Could you check a few things on this model? Use its own coordinates, in mm. Face numbers are marked on the shaded views. A direction names the side the tool comes from. Coordinates: 2 decimals unless noted, no trailing zeros. Loops run counter-clockwise (first coordinate to the right, second up) from the corner with the lowest first, then second, coordinate; pieces in that order, holes last. Notation, with made-up numbers: (13, -24.75) -> (24, -24.75) arc R23 cw to (24, 1.25) -> close; hole circle Ø1 at (86.25, 65.25). An arc over 180 degrees is marked (long way). One line per question, with ' | ' between items.
```python
from build123d import *

# Parameters (mm, degrees)
ESQUISSE1_R             = 16
BOSS_EXTRU_1_DEPTH      = 36.4
ESQUISSE2_R             = 9.5
BOSS_EXTRU_2_DEPTH      = 2.25
ESQUISSE3_R             = 4
BOSS_EXTRU_3_DEPTH      = 2.6
ESQUISSE4_R             = 3
BOSS_EXTRU_4_DEPTH      = 16.15
ESQUISSE5_R             = 1.5
ENL_V_MAT_EXTRU_1_DEPTH = 3.8


with BuildPart() as part:
    # Esquisse1 → Boss.-Extru.1 (new body)
    with BuildSketch(Plane.XY):
        Circle(ESQUISSE1_R)
    extrude(amount=BOSS_EXTRU_1_DEPTH)

    # Esquisse2 → Boss.-Extru.2 (add)
    with BuildSketch(Plane.XY.offset(36.4)):
        Circle(ESQUISSE2_R)
    extrude(amount=BOSS_EXTRU_2_DEPTH)

    # Esquisse3 → Boss.-Extru.3 (add)
    with BuildSketch(Plane.XY.offset(38.65)):
        Circle(ESQUISSE3_R)
    extrude(amount=BOSS_EXTRU_3_DEPTH)

    # Esquisse4 → Boss.-Extru.4 (add)
    with BuildSketch(Plane.XY.offset(41.25)):
        Circle(ESQUISSE4_R)
    extrude(amount=BOSS_EXTRU_4_DEPTH)

    # Esquisse5 → Enlèv. mat.-Extru.1 (cut)
    with BuildSketch(Plane.XY.offset(36.4)):
        with Locations((0, 13)):
            Circle(ESQUISSE5_R)
        with Locations((13, 0)):
            Circle(ESQUISSE5_R)
        with Locations((0, -13)):
            Circle(ESQUISSE5_R)
        with Locations((-13, 0)):
            Circle(ESQUISSE5_R)
    extrude(amount=-ENL_V_MAT_EXTRU_1_DEPTH, mode=Mode.SUBTRACT)


solid = part.part
```
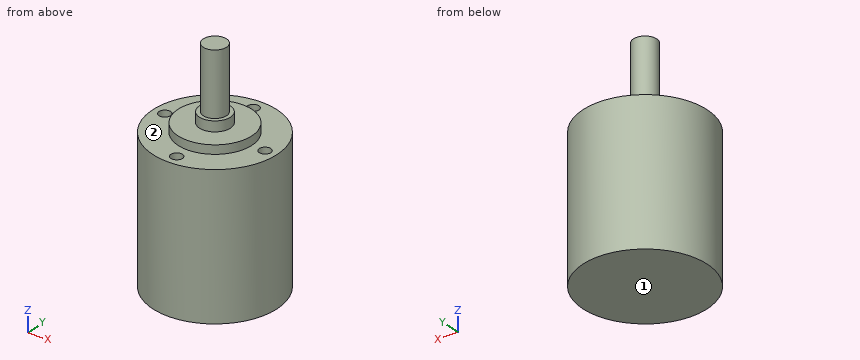
Q1. Imagine slicing it at C-C on z = 4. Write out the boundary of the cut face in (x, y).
Values follow:
outline: circle Ø32 at (0, 0)
Q2. Please list where these lines run through material, in increasing order: L1, parallel to Y at x = 0, z = 35; L2, parallel to Z at x = -13, y = -1; L3, parallel to Z at x = -2.5, y = -11.5. Write a range as [from, to].
Values follow:
L1: y = [-16, -14.5], [-11.5, 11.5], [14.5, 16] | L2: z = [0, 32.6] | L3: z = [0, 36.4]
Q3. For the marked faces 1 and 2, which set-ups out of +Z, -Z, +X, -X, +Y, -Y let a thin tool reach every point of the face, with its end or its side?
Values follow:
face 1: -Z, +X, -X, +Y, -Y | face 2: +Z
Q4. Imagine slicing it at A-A on y = 8. Write out the boundary of the cut face in (x, z).
Values follow:
outline: (-13.86, 0) -> (13.86, 0) -> (13.86, 36.4) -> (5.12, 36.4) -> (5.12, 38.65) -> (-5.12, 38.65) -> (-5.12, 36.4) -> (-13.86, 36.4) -> close
Q5. Imagine slicing it at B-B on x = 0. Write out the boundary of the cut face in (y, z), plus the area to 3 significant figures.
Values follow:
outline: (-16, 0) -> (16, 0) -> (16, 36.4) -> (14.5, 36.4) -> (14.5, 32.6) -> (11.5, 32.6) -> (11.5, 36.4) -> (9.5, 36.4) -> (9.5, 38.65) -> (4, 38.65) -> (4, 41.25) -> (3, 41.25) -> (3, 57.4) -> (-3, 57.4) -> (-3, 41.25) -> (-4, 41.25) -> (-4, 38.65) -> (-9.5, 38.65) -> (-9.5, 36.4) -> (-11.5, 36.4) -> (-11.5, 32.6) -> (-14.5, 32.6) -> (-14.5, 36.4) -> (-16, 36.4) -> close | area: 1,300 mm2
Q6. For pin 1 (1.8 mm diameter, centred on x = -13, y = 0, fed in from +Z); pin 2 (3.5 mm diameter, centred on x = -13, y = -0.5, fed in from +Z); pin 3 (6 mm diameter, centred on x = -6, y = -10, fed in from +Z); pin 4 (8 mm diameter, centred on y = -11.5, z = 44.5, fed in from -X), each with a flat end and sliding along its axis, tell me the tip position at first contact or that it passes through.
Values follow:
pin 1: stops at z = 32.6 | pin 2: stops at z = 36.4 | pin 3: stops at z = 38.65 | pin 4: passes through
